Could you check a few things on this model? Use its own coordinates, in mm. Face numbers are marked on the shaded views. A direction names the side the tool comes from. Round coordinates to 2 decimals unless told otherwise and drop trailing zeros. Loops run counter-clockwise (first coordinate to the right, second up) from the corner with the lowest first, then second, coordinate; pieces in that order, holes last.
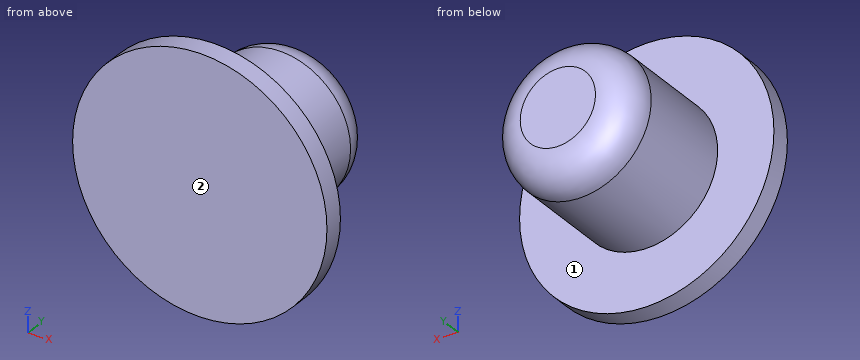
from build123d import *

# Parameters (mm, degrees)
SKETCH1_R           = 19.1
SKETCH1_R_2         = 10.65
BOSS_EXTRUDE1_DEPTH = 3
SKETCH1_2_R         = 10.65
BOSS_EXTRUDE2_DEPTH = 22.8
FILLET1_R           = 5


with BuildPart() as part:
    # Sketch1 → Boss-Extrude1 (new body)
    with BuildSketch(Plane(origin=(0, 0, 0), x_dir=(1, 0, 0), z_dir=(0, 1, 0))):
        Circle(SKETCH1_R)
        Circle(SKETCH1_R_2, mode=Mode.SUBTRACT)
    extrude(amount=BOSS_EXTRUDE1_DEPTH)

    # Sketch1<2> → Boss-Extrude2 (add)
    with BuildSketch(Plane(origin=(0, 0, 0), x_dir=(1, 0, 0), z_dir=(0, 1, 0))):
        Circle(SKETCH1_2_R)
    extrude(amount=BOSS_EXTRUDE2_DEPTH)

    # Fillet1
    fillet1_edges = [part.edges().sort_by_distance(p)[0] for p in [
        (-10.65, 22.8, 0),
    ]]
    fillet(fillet1_edges, radius=FILLET1_R)


solid = part.part
Item 1: For the marked faces 1 and 2, which set-ups out of +Z, -Z, +X, -X, +Y, -Y let a thin tool reach every point of the face, with its end or its side?
Results list:
face 1: +Y
face 2: +Z, -Z, +X, -X, -Y
Item 2: If we section it at A-A, the plane z = 0: Please give me the cut outline in (x, y).
Results list:
outline: (-19.1, 0) - (19.1, 0) - (19.1, 3) - (10.65, 3) - (10.65, 17.8) arc R5 ccw to (5.65, 22.8) - (-5.65, 22.8) arc R5 ccw to (-10.65, 17.8) - (-10.65, 3) - (-19.1, 3) - close
Item 3: Will these pins go through, and if not, where does the flat tip stop? pin 1 (3 mm diameter, centred on y = 17, z = -6.5, fed in from +X); pin 2 (12 mm diameter, centred on y = 10.5, z = 3, fed in from -X); pin 3 (3 mm diameter, centred on y = 3.5, z = -8, fed in from +X).
Results list:
pin 1: stops at x = 9.4
pin 2: stops at x = -10.65
pin 3: stops at x = 17.93
Item 4: If we section it at C-C, the plane y = 8: Please give me the cut outline in (x, z).
Results list:
outline: circle Ø21.3 at (0, 0)
Item 5: If we section it at D-D, the plane z = -14.5: Please give me the cut outline in (x, y).
Results list:
outline: (-12.43, 0) - (12.43, 0) - (12.43, 3) - (-12.43, 3) - close
Item 6: If we section it at B-B, the plane x = 0: Please give me the cut outline in (y, z), then the cut area to 3 significant figures.
Results list:
outline: (0, -19.1) - (3, -19.1) - (3, -10.65) - (17.8, -10.65) arc R5 ccw to (22.8, -5.65) - (22.8, 5.65) arc R5 ccw to (17.8, 10.65) - (3, 10.65) - (3, 19.1) - (0, 19.1) - close
area: 526 mm2
Item 7: If I drill on line 1 along Y through (x, z) = (12, -4); line 2 along Z through (x, y) = (1, 15.25); line 3 along Z through (x, y) = (8.5, 21.25), over which ranges is the centre line in solid material (lowest first)?
Results list:
line 1: y = 0 to 3
line 2: z = -10.6 to 10.6
line 3: z = -3.7 to 3.7
